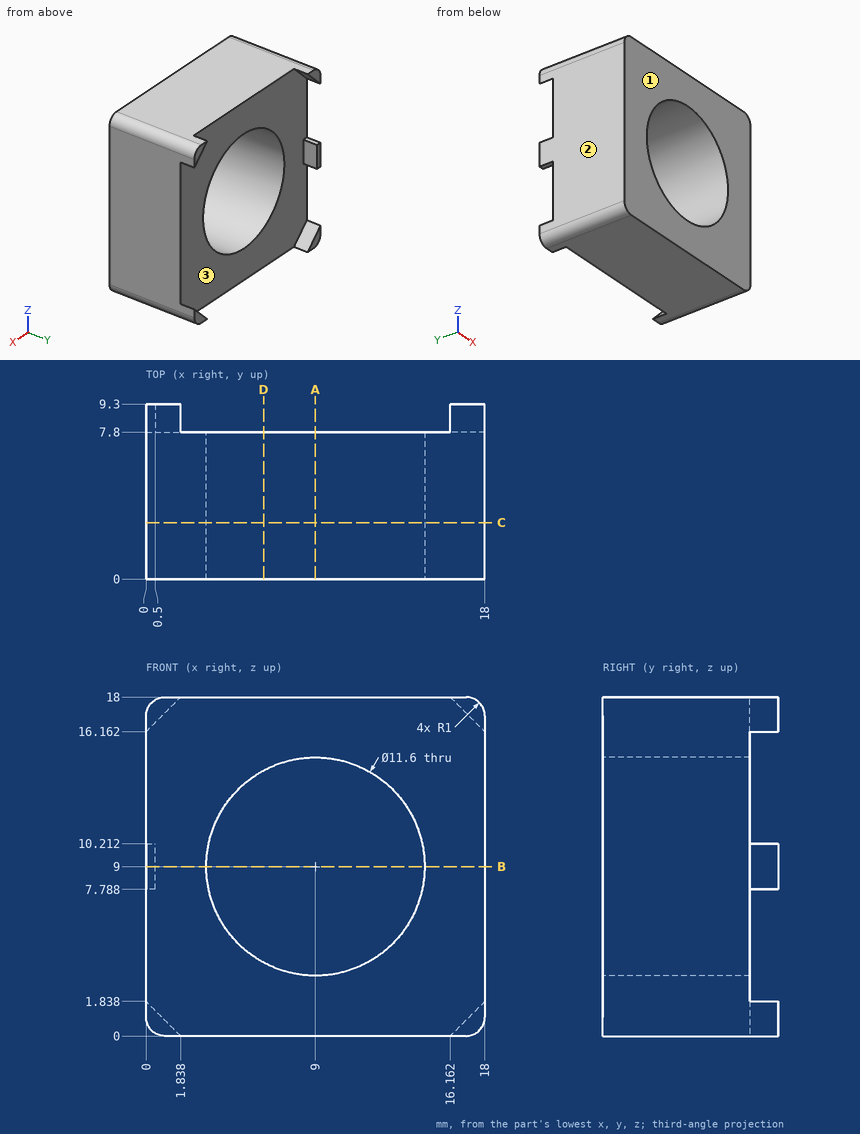
Drawing for the job (mm, zero at the part's lowest x, y, z). Round coordinates to 2 decimals unless told otherwise and drop trailing zeros. Loops run counter-clockwise (first coordinate to the right, second up) from the corner with the lowest first, then second, coordinate; pieces in that order, holes last. Notation, with made-up numbers: (20, -38.75) - (30, -38.75) arc R17 ccw to (30, -20.75) - close; hole circle Ø2 at (-27, -8.5). An arc over 180 degrees is marked (long way). Return JSON: item names as keys, results as strings. Group by question number.
Q1. Band-saw the part on B-B on z = 9. Give the cut face in (x, y).
Q2. Band-saw the part on C-C on y = 3. Give the cut face in (x, z).
Q3. Two-plate mould, pull along X, no slides. Class the marked faces 1, 2 and 3: +X half, -X half, draft (parallel to the pull), parting line (faces both ways), or undercut.
Q4. Band-saw the part on D-D on x = 6.25. Give the cut face in (y, z).
Q5. Drill centre lines: line 1 along Z through (x, y) = (9, 2.25); line 2 along Y through (x, z) = (3, 8.25); line 3 along X through (y, z) = (2, 8). Where is each one in solid material? Low to high. Write a range as [from, to].
Q6. Flat gauge pins, fed straight in: pin 1 Ø6 at (x, z) = (16, 12.5) entering from +Y; pin 2 Ø0.8 at (y, z) = (8.5, 9.5) entering from +X; pin 3 Ø10.5 at (x, z) = (9, 9) entering from +Y. Where does each tip first touch, or does it go through?
Q7. Band-saw the part on A-A on x = 9. Give the cut face in (y, z).
Solutions:
{
 "1": {"outline": "(0, 0) - (3.2, 0) - (3.2, 7.8) - (0.5, 7.8) - (0.5, 9.3) - (0, 9.3) - close; (14.8, 0) - (18, 0) - (18, 7.8) - (14.8, 7.8) - close"},
 "2": {"outline": "(0, 1) arc R1 ccw to (1, 0) - (17, 0) arc R1 ccw to (18, 1) - (18, 17) arc R1 ccw to (17, 18) - (1, 18) arc R1 ccw to (0, 17) - close; hole circle Ø11.6 at (9, 9)"},
 "3": {"face 1": "draft", "face 2": "-X half", "face 3": "undercut"},
 "4": {"outline": "(0, 0) - (7.8, 0) - (7.8, 3.89) - (0, 3.89) - close; (0, 14.11) - (7.8, 14.11) - (7.8, 18) - (0, 18) - close"},
 "5": {"line 1": "z = [0, 3.2], [14.8, 18]", "line 2": "y = [0, 7.8]", "line 3": "x = [0, 3.29], [14.71, 18]"},
 "6": {"pin 1": "stops at y = 7.8", "pin 2": "stops at x = 0.5", "pin 3": "passes through"},
 "7": {"outline": "(0, 0) - (7.8, 0) - (7.8, 3.2) - (0, 3.2) - close; (0, 14.8) - (7.8, 14.8) - (7.8, 18) - (0, 18) - close"}
}
